```python
from build123d import *

# Parameters (mm, degrees)
BOSS_EXTRUDE1_DEPTH = 6.35
SKETCH20_R          = 35
BOSS_EXTRUDE5_DEPTH = 19.05
CUT_EXTRUDE14_DEPTH = 103.562956276
CHAMFER1_SIZE       = 19.05
SKETCH22_R          = 3.175
CUT_EXTRUDE15_DEPTH = 109.709596838
SKETCH24_R          = 5
CUT_EXTRUDE16_DEPTH = 114.565219549
SKETCH25_R          = 2.38125
CUT_EXTRUDE17_DEPTH = 10
CUT_EXTRUDE18_DEPTH = 10
CHAMFER2_SIZE       = 2.5
FILLET1_R           = 1.5875


with BuildPart() as part:
    # Sketch1 → Boss-Extrude1 (new body)
    with BuildSketch(Plane(origin=(0, 0, 0), x_dir=(0, 0, -1), z_dir=(1, 0, 0))):
        with BuildLine():
            Line((-34.741931963, -4.242424242), (-26.800918943, -69.272727273))
            ThreePointArc((-26.800918943, -69.272727273), (0, -93), (26.800918943, -69.272727273))
            Line((26.800918943, -69.272727273), (34.741931963, -4.242424242))
            ThreePointArc((34.741931963, -4.242424242), (0, 35), (-34.741931963, -4.242424242))
        make_face()
        Polygon((4.353205728, 11.960334439), (-11.960334439, 4.353205728), (-4.353205728, -11.960334439), (11.960334439, -4.353205728), align=None, mode=Mode.SUBTRACT)
    extrude(amount=BOSS_EXTRUDE1_DEPTH)

    # Sketch20 → Boss-Extrude5 (add)
    with BuildSketch(Plane(origin=(6.35, 0, 0), x_dir=(0, 0, -1), z_dir=(1, 0, 0))):
        with Locations(Location((0, 0, 0), (0, 0, 186.962062691))):
            Circle(SKETCH20_R)
    extrude(amount=BOSS_EXTRUDE5_DEPTH)

    # Sketch21 → Cut-Extrude14 (cut, through all)
    with BuildSketch(Plane.ZY):
        Polygon((-19.067760927, 15.897892729), (-24.435012851, 4.387783834), (-10.840396045, -1.951490092), (-5.473144121, 9.558618803), align=None)
        Polygon((-11.960334439, -4.353205728), (-4.353205728, 11.960334439), (11.960334439, 4.353205728), (4.353205728, -11.960334439), align=None)
        Polygon((10.840396045, 1.951490092), (5.473144121, -9.558618803), (19.067760927, -15.897892729), (24.435012851, -4.387783834), align=None)
    extrude(amount=-CUT_EXTRUDE14_DEPTH, mode=Mode.SUBTRACT)

    # Chamfer1
    # the kernel refuses this chamfer: 19.05 mm, written as the material it takes off along each edge
    with BuildSketch(Plane(origin=(25.4, 0, 0), x_dir=(0, -0.1212121212106579, 0.9926266275249788), z_dir=(0, 0.9926266275249788, 0.1212121212106579))) as chamfer1_piece_1:
        Polygon((35, -CHAMFER1_SIZE), (35 - CHAMFER1_SIZE, 0), (35, 0), align=None)
    revolve(axis=Axis((25.4, 0, 0), (1, 0, 0)), mode=Mode.SUBTRACT)

    # Sketch22 → Cut-Extrude15 (cut, through all)
    with BuildSketch(Plane(origin=(0, 5.755054448, 2.683625962), x_dir=(-1, 0, 0), z_dir=(0, -0.9063077870366495, -0.4226182617407006))):
        with Locations(Location((-13.4, -16.5, 0), (0, 0, 90))):
            Circle(SKETCH22_R)
    cut_extrude15 = extrude(amount=-CUT_EXTRUDE15_DEPTH, mode=Mode.SUBTRACT)

    # Sketch24 → Cut-Extrude16 (cut, through all)
    with BuildSketch(Plane(origin=(0, 10.286593383, 4.796717271), x_dir=(-1, 0, 0), z_dir=(0, -0.9063077870366495, -0.4226182617407006))):
        with Locations(Location((-13.4, -16.5, 0), (0, 0, 90))):
            Circle(SKETCH24_R)
    cut_extrude16 = extrude(amount=-CUT_EXTRUDE16_DEPTH, mode=Mode.SUBTRACT)

    # Sketch25 → Cut-Extrude17 (cut)
    with BuildSketch(Plane(origin=(0, -5.755054448, -2.683625962), x_dir=(1, 0, 0), z_dir=(0, 0.9063077870366495, 0.4226182617407006))):
        with Locations(Location((13.4, -16.5, 0), (0, 0, 270))):
            Circle(SKETCH25_R)
    cut_extrude17 = extrude(amount=-CUT_EXTRUDE17_DEPTH, mode=Mode.SUBTRACT)

    # Mirror1: Cut-Extrude15, Cut-Extrude16, Cut-Extrude17 across plane
    add(cut_extrude15.mirror(Plane(origin=(0, 0, 0), x_dir=(1, 0, 0), z_dir=(0, 0.422618261740701, -0.9063077870366492))), mode=Mode.SUBTRACT)
    add(cut_extrude16.mirror(Plane(origin=(0, 0, 0), x_dir=(1, 0, 0), z_dir=(0, 0.422618261740701, -0.9063077870366492))), mode=Mode.SUBTRACT)
    add(cut_extrude17.mirror(Plane(origin=(0, 0, 0), x_dir=(1, 0, 0), z_dir=(0, 0.422618261740701, -0.9063077870366492))), mode=Mode.SUBTRACT)

    # Sketch19 → Cut-Extrude18 (cut)
    with BuildSketch(Plane(origin=(6.35, 0, 0), x_dir=(0, 0, -1), z_dir=(1, 0, 0))):
        with BuildLine():
            Line((13.556349186, -44.768650814), (13.556349186, -49.768650814))
            ThreePointArc((13.556349186, -49.768650814), (15.556349186, -51.768650814), (17.556349186, -49.768650814))
            Line((17.556349186, -49.768650814), (17.556349186, -44.768650814))
            ThreePointArc((17.556349186, -44.768650814), (15.556349186, -42.768650814), (13.556349186, -44.768650814))
        make_face()
        with BuildLine():
            Line((-10, -60.325), (-10, -65.325))
            ThreePointArc((-10, -65.325), (0, -75.325), (10, -65.325))
            Line((10, -65.325), (10, -60.325))
            ThreePointArc((10, -60.325), (0, -50.325), (-10, -60.325))
        make_face()
        with BuildLine():
            Line((17.556349186, -80.881349186), (17.556349186, -75.881349186))
            ThreePointArc((17.556349186, -75.881349186), (15.556349186, -73.881349186), (13.556349186, -75.881349186))
            Line((13.556349186, -75.881349186), (13.556349186, -80.881349186))
            ThreePointArc((13.556349186, -80.881349186), (15.556349186, -82.881349186), (17.556349186, -80.881349186))
        make_face()
        with BuildLine():
            Line((-17.556349186, -44.768650814), (-17.556349186, -49.768650814))
            ThreePointArc((-17.556349186, -49.768650814), (-15.556349186, -51.768650814), (-13.556349186, -49.768650814))
            Line((-13.556349186, -49.768650814), (-13.556349186, -44.768650814))
            ThreePointArc((-13.556349186, -44.768650814), (-15.556349186, -42.768650814), (-17.556349186, -44.768650814))
        make_face()
        with BuildLine():
            Line((-13.556349186, -80.881349186), (-13.556349186, -75.881349186))
            ThreePointArc((-13.556349186, -75.881349186), (-15.556349186, -73.881349186), (-17.556349186, -75.881349186))
            Line((-17.556349186, -75.881349186), (-17.556349186, -80.881349186))
            ThreePointArc((-17.556349186, -80.881349186), (-15.556349186, -82.881349186), (-13.556349186, -80.881349186))
        make_face()
    extrude(amount=-CUT_EXTRUDE18_DEPTH, mode=Mode.SUBTRACT)


with BuildPart() as body_2:
    # Mirror2: mirrored copy
    add(part.part.mirror(Plane(origin=(0, 0, 0), x_dir=(0, 0, 1), z_dir=(1, 0, 0))))


with BuildPart() as part_1:
    add(part.part)

    # Chamfer2
    chamfer2_edges = [part_1.edges().sort_by_distance(p)[0] for p in [
        (0, -47.268650814, 13.556349186),
        (0, -42.768650814, 15.556349186),
        (0, -47.268650814, 17.556349186),
        (0, -51.768650814, 15.556349186),
        (0, -47.268650814, -17.556349186),
        (0, -42.768650814, -15.556349186),
        (0, -47.268650814, -13.556349186),
        (0, -51.768650814, -15.556349186),
    ]]
    chamfer(chamfer2_edges, length=CHAMFER2_SIZE)

    # Fillet1
    fillet1_edges = [part_1.edges().sort_by_distance(p)[0] for p in [
        (12.7, -4.353205728, -11.960334439),
        (8.262078305, 4.387783834, -24.435012851),
        (12.7, 11.960334439, -4.353205728),
        (8.262078305, 15.897892729, -19.067760927),
        (8.262078305, -4.387783834, 24.435012851),
        (12.7, 4.353205728, 11.960334439),
        (12.7, -11.960334439, 4.353205728),
        (8.262078305, -15.897892729, 19.067760927),
    ]]
    fillet(fillet1_edges, radius=FILLET1_R)


solid = part_1.part
```
Geometry: final body of the model. Coordinates: model frame, mm. A direction names the side the tool comes from. Give positions to 0.01 mm unless a question says otherwise; leave off trailing zeros. Use CSV: the item, a comma, the result in double quotes.
(1) Ray query, line 1 along Y through (x, z) = (6, 16.5); line 2 along Y through (x, z) = (4.5, 1); line 3 along X through (y, z) = (-70.5, 18). Return the intervals inside material, ascending. Write a range as [from, to].
From the geometry:
line 1,"[-87.37, -82.64], [-74.12, -51.53], [-43.01, -14.7], [-0.69, 30.87]"
line 2,"[-92.98, -75.27], [-50.38, -10.4], [9.46, 34.99]"
line 3,"[0, 6.35]"
(2) Pull-direction query (Z, two-part tool) for faces 4 (the face through (3.131, -37.213, -30.716)), 5 (the face through (3, -63, -10)), 6 (the face through (3.13, 34.99, -0.83)); classes: released by +Z, released by -Z, zero draft, split by the parting line, or undercut.
From the geometry:
face 4,"released by -Z"
face 5,"undercut"
face 6,"split by the parting line"
(3) First-contact query: P1, Ø4, axis at x = 2, y = -63, coming from the -Z side; P2, Ø5.5, axis at x = 1.5, y = -78, coming from the -Z side; P3, Ø4, axis at x = 2.5, y = -77.5, coming from the +Z side; P4, Ø8, axis at y = 11, z = -17.5, coming from the -X side. Flat tips, straight axial feed; report the tip coordinate or a pass-through.
From the geometry:
P1,"z = -27.81"
P2,"z = -25.37"
P3,"z = 25.27"
P4,"x = 0"
(4) Access query for faces 1 (the face through (4, -47, 17.556)), 2 (the face through (13.43, -7.86, -21.83)), 3 (the face through (1.232, -47.234, -12.289)). Directions: +Z, -Z, +X, -X, +Y, -Y. A direction counts if a zero-diameter tool reaches every point of the face in a straight line with its end or side. Return the directions, or none.
From the geometry:
face 1,"+X, -X"
face 2,"none"
face 3,"-X"
